from build123d import *

# Parameters (mm, degrees)
SKETCH_1_W      = 36
SKETCH_1_H      = 36
EXTRUDE_1_DEPTH = 11
FILLET_1_R      = 1
SKETCH_2_W      = 25
SKETCH_2_H      = 25
EXTRUDE_2_DEPTH = 5
FILLET_2_R      = 1
SKETCH_3_R      = 7.5
EXTRUDE_3_DEPTH = 10
SKETCH_4_R      = 10
EXTRUDE_4_DEPTH = 5
FILLET_3_R      = 1


with BuildPart() as part:
    # 草图1 → 凸台-拉伸1 (new body)
    with BuildSketch(Plane.XY):
        with Locations((18, -18)):
            Rectangle(SKETCH_1_W, SKETCH_1_H)
    extrude(amount=EXTRUDE_1_DEPTH)

    # 圆角1
    fillet_1_edges = [part.edges().sort_by_distance(p)[0] for p in [
        (36, -18, 11),
        (18, 0, 11),
        (0, -18, 11),
        (18, 0, 0),
        (36, -18, 0),
        (18, -36, 0),
        (0, -18, 0),
        (0, 0, 5.5),
        (36, 0, 5.5),
        (36, -36, 5.5),
        (0, -36, 5.5),
        (18, -36, 11),
    ]]
    fillet(fillet_1_edges, radius=FILLET_1_R)

    # 草图2 → 凸台-拉伸2 (add)
    with BuildSketch(Plane.XY.offset(11)):
        with Locations((18, -18)):
            Rectangle(SKETCH_2_W, SKETCH_2_H)
    extrude(amount=EXTRUDE_2_DEPTH)

    # 圆角2
    fillet_2_edges = [part.edges().sort_by_distance(p)[0] for p in [
        (5.5, -5.5, 13.5),
        (5.5, -30.5, 13.5),
        (30.5, -30.5, 13.5),
        (30.5, -5.5, 13.5),
        (5.5, -18, 16),
        (18, -30.5, 16),
        (30.5, -18, 16),
        (18, -5.5, 16),
    ]]
    fillet(fillet_2_edges, radius=FILLET_2_R)

    # 草图3 → 凸台-拉伸3 (add)
    with BuildSketch(Plane.XY.offset(16)):
        with Locations((18, -18)):
            Circle(SKETCH_3_R)
    extrude(amount=EXTRUDE_3_DEPTH)

    # 草图4 → 凸台-拉伸4 (add)
    with BuildSketch(Plane.XY.offset(26)):
        with Locations((18, -18)):
            Circle(SKETCH_4_R)
    extrude(amount=EXTRUDE_4_DEPTH)

    # 圆角3
    fillet_3_edges = [part.edges().sort_by_distance(p)[0] for p in [
        (10.5, -18, 26),
        (8, -18, 26),
        (8, -18, 31),
    ]]
    fillet(fillet_3_edges, radius=FILLET_3_R)


solid = part.part
Source: CAD feature listing. Evaluate the final solid. Frame: model axes, mm. A direction names the side the tool comes from. Coordinates: 2 decimals unless noted, no trailing zeros. Loops run counter-clockwise (first coordinate to the right, second up) from the corner with the lowest first, then second, coordinate; pieces in that order, holes last. Notation, with made-up numbers: (88, -21) -> (122, -21) arc R8 ccw to (122, -10) -> close; hole circle Ø3 at (46, 42). An arc over 180 degrees is marked (long way). Answer in a Markdown table with one row per item. Add a question column.
Q1. Section B-B on x = 18. Return the cut outline in (y, z), and give its area (3 significant figures).
Q2. Section C-C on z = 23. Return the cut outline in (x, y).
Q3. Reachability of faces 4 (the face through (30.199, -30.215, 13.028)), 5 (the face through (21.3, -26, 26)), 6 (the face through (5.801, -30.215, 13.028)), 7 (the face through (5.5, -18, 13)) from +Z, -Z, +X, -X, +Y, -Y: full face, straight path, thin tool, end or side. Return the list, or none.
Q4. Ray query, line 1 along Z through (x, y) = (34, -22.5); line 2 along Z through (x, y) = (8, -13.5); line 3 along Y through (x, z) = (17, 14.5). Return the intervals inside material, ascending.
Q5. Section D-D on y = -32. Return the cut outline in (x, z).
Q6. Pull-direction query (Z, two-part tool) for faces 1 (the face through (5.801, -5.785, 13.028)), 2 (the face through (18, -10, 16)), 3 (the face through (18.161, -5.785, 15.699)); classes: pulls with the +Z half, pulls with the -Z half, needs draft (parallel to the pull), parting line crosses it, or undercut.
Q7. Contact query for flat-ended pins moving along their axis: pin 1 Ø3 at (x, z) = (18, 12) entering from -Y; pin 2 Ø8 at (x, z) = (19.5, 24) entering from -Y; pin 3 Ø5 at (y, z) = (-19.5, 12) entering from +X; pin 4 Ø3 at (y, z) = (-19, 13) entering from +X. Output: stop coordinate, or through.
Q8. Section A-A on y = -18. Return the cut outline in (x, z), and give its area (3 significant figures).
Computed values:
| question | item | result |
|---|---|---|
| 1 | outline | (-36, 1) arc R1 ccw to (-35, 0) -> (-1, 0) arc R1 ccw to (0, 1) -> (0, 10) arc R1 ccw to (-1, 11) -> (-5.5, 11) -> (-5.5, 15) arc R1 ccw to (-6.5, 16) -> (-10.5, 16) -> (-10.5, 25) arc R1 cw to (-9.5, 26) -> (-9, 26) arc R1 ccw to (-8, 27) -> (-8, 30) arc R1 ccw to (-9, 31) -> (-27, 31) arc R1 ccw to (-28, 30) -> (-28, 27) arc R1 ccw to (-27, 26) -> (-26.5, 26) arc R1 cw to (-25.5, 25) -> (-25.5, 16) -> (-29.5, 16) arc R1 ccw to (-30.5, 15) -> (-30.5, 11) -> (-35, 11) arc R1 ccw to (-36, 10) -> close |
| 1 | area | 769 mm^2 |
| 2 | outline | circle Ø15 at (18, -18) |
| 3 | face 4 | +Z, +X, -Y |
| 3 | face 5 | none |
| 3 | face 6 | +Z, -X, -Y |
| 3 | face 7 | +Z, -X, +Y, -Y |
| 4 | line 1 | z = 0 to 11 |
| 4 | line 2 | z = 0 to 16 |
| 4 | line 3 | y = -30.5 to -5.5 |
| 5 | outline | (0, 1) arc R1 ccw to (1, 0) -> (35, 0) arc R1 ccw to (36, 1) -> (36, 10) arc R1 ccw to (35, 11) -> (1, 11) arc R1 ccw to (0, 10) -> close |
| 6 | face 1 | needs draft |
| 6 | face 2 | undercut |
| 6 | face 3 | pulls with the +Z half |
| 7 | pin 1 | stops at y = -35.87 |
| 7 | pin 2 | stops at y = -28 |
| 7 | pin 3 | stops at x = 36 |
| 7 | pin 4 | stops at x = 30.5 |
| 8 | outline | (0, 1) arc R1 ccw to (1, 0) -> (35, 0) arc R1 ccw to (36, 1) -> (36, 10) arc R1 ccw to (35, 11) -> (30.5, 11) -> (30.5, 15) arc R1 ccw to (29.5, 16) -> (25.5, 16) -> (25.5, 25) arc R1 cw to (26.5, 26) -> (27, 26) arc R1 ccw to (28, 27) -> (28, 30) arc R1 ccw to (27, 31) -> (9, 31) arc R1 ccw to (8, 30) -> (8, 27) arc R1 ccw to (9, 26) -> (9.5, 26) arc R1 cw to (10.5, 25) -> (10.5, 16) -> (6.5, 16) arc R1 ccw to (5.5, 15) -> (5.5, 11) -> (1, 11) arc R1 ccw to (0, 10) -> close |
| 8 | area | 769 mm^2 |
